```python
from build123d import *

# Parameters (mm, degrees)
IZIM1_R                     = 2.187508585
Y_KSEKLIK_EKSTR_ZYON1_DEPTH = 177
RADYUS1_R                   = 1
IZIM2_W                     = 5.115236905
IZIM2_H                     = 5.042987796
Y_KSEKLIK_EKSTR_ZYON2_DEPTH = 5
Y_KSEKLIK_EKSTR_ZYON3_DEPTH = 2.5
IZIM4_W                     = 9.955982426
IZIM4_H                     = 3.788849983
KES_EKSTR_ZYON1_DEPTH       = 5
IZIM5_R                     = 0.420224292
Y_KSEKLIK_EKSTR_ZYON4_DEPTH = 5


with BuildPart() as part:
    # Çizim1 → Yükseklik-Ekstrüzyon1 (new body)
    with BuildSketch(Plane(origin=(0, 0, 0), x_dir=(1, 0, 0), z_dir=(0, 1, 0))):
        Circle(IZIM1_R)
    extrude(amount=Y_KSEKLIK_EKSTR_ZYON1_DEPTH)

    # Radyus1
    radyus1_edges = [part.edges().sort_by_distance(p)[0] for p in [
        (-2.187508585, 0, 0),
    ]]
    fillet(radyus1_edges, radius=RADYUS1_R)

    # Çizim2 → Yükseklik-Ekstrüzyon2 (add)
    with BuildSketch(Plane(origin=(0, 177, 0), x_dir=(1, 0, 0), z_dir=(0, 1, 0))):
        with Locations((-0.108373663, 0.052171697)):
            Rectangle(IZIM2_W, IZIM2_H)
    extrude(amount=-Y_KSEKLIK_EKSTR_ZYON2_DEPTH)

    # Çizim3 → Yükseklik-Ekstrüzyon3 (add, symmetric)
    with BuildSketch(Plane.XY):
        with BuildLine():
            Line((0, 176.935410542), (7.547644812, 176.935410542))
            ThreePointArc((7.547644812, 176.935410542), (9.98246541, 174.500589945), (7.547644812, 172.065769347))
            Line((7.547644812, 172.065769347), (0, 172.065769347))
            ThreePointArc((0, 172.065769347), (-2.434820598, 174.500589945), (0, 176.935410542))
        make_face()
    extrude(amount=Y_KSEKLIK_EKSTR_ZYON3_DEPTH, both=True)

    # Çizim4 → Kes-Ekstrüzyon1 (cut)
    with BuildSketch(Plane(origin=(0, 176.935410542, 0), x_dir=(1, 0, 0), z_dir=(0, 1, 0))):
        with Locations((8.319846031, 0.078445098)):
            Rectangle(IZIM4_W, IZIM4_H)
    extrude(amount=-KES_EKSTR_ZYON1_DEPTH, mode=Mode.SUBTRACT)

    # Çizim5 → Yükseklik-Ekstrüzyon4 (add)
    with BuildSketch(Plane.XY.offset(2.5)):
        with Locations((7.702816728, 174.562062813)):
            Circle(IZIM5_R)
    extrude(amount=-Y_KSEKLIK_EKSTR_ZYON4_DEPTH)


solid = part.part
```
Design review of the part built by this model. Coordinates are the model's own, in mm. Give positions to 0.01 mm unless a question says otherwise; leave off trailing zeros. Order: outer loops, then holes, each group sorted by start corner. A loop starts at its lowest first (then second) coordinate and runs counter-clockwise, first axis right, second up. Notation, with made-up numbers: M 42,17 L 74,17 A23 cw 74,30 Z; hole C 15,78.5 d4. An arc over 180 degrees is marked long. One line per question, with ' | ' between items. Start each with the question number.
Q1. We need section B-B (y = 67.5). Write out the cut boundary in (x, z).
Q2. For pin 1 Ø3 at (x, z) = (7.5, 1.5) entering from -Y; pin 2 Ø2 at (x, y) = (0, 111.5) entering from -Z; pin 3 Ø1.5 at (x, y) = (5, 173.5) entering from -Z, all flat-tipped, find the tip position at first contact; note any pin that passes through.
Q3. We need section A-A (z = 0). Write out the cut boundary in (x, y).
Q4. For L1, parallel to Z at x = 0, y = 168.5; L2, parallel to Y at x = 1.5, z = -0.9, list the stretches that pass through material, from the lowest coordinate up. Write a range as [from, to].
Q5. The part is to be moulded in two halves that separate along Z. For faces 1 (the face through (7, 175, 1.816)), 2 (the face through (0, 175, -2.574)), 3 (the face through (3, 172.066, 0)), say which applies: +Z half, -Z half, draft (parallel to the pull), parting line (faces both ways), or undercut.
Returned:
1) outline: C 0,0 d4.38
2) pin 1: y = 172.07 | pin 2: z = -2.19 | pin 3: z = -2.5
3) outline: M -2.67,172 L -2.19,172 L -2.19,1 A1 ccw -1.19,0 L 1.19,0 A1 ccw 2.19,1 L 2.19,172 L 2.45,172 L 2.45,172.07 L 3.34,172.07 L 3.34,176.94 L 2.45,176.94 L 2.45,177 L -2.67,177 Z; C 7.7,174.56 d0.84
4) L1: [-2.19, 2.19] | L2: [0.17, 177]
5) face 1: undercut | face 2: -Z half | face 3: draft
